Could you check a few things on this model? Use its own coordinates, in mm. Face numbers are marked on the shaded views. A direction names the side the tool comes from. Give positions to 0.01 mm unless a question says otherwise; leave off trailing zeros. Loops run counter-clockwise (first coordinate to the right, second up) from the corner with the lowest first, then second, coordinate; pieces in that order, holes last. Notation, with made-up numbers: (67, 57) - (96, 57) arc R21 ccw to (96, 96) - close; hole circle Ø7 at (39.25, 13). An arc over 180 degrees is marked (long way). Write each question's results on one line, items separated by ' | '. Start each with the question number.
(1) Suppose I cut it at B-B (y = 0). Please give me the cut outline in (x, z), and give its area (3 significant figures).
(2) Suppose I cut it at C-C (x = 43). Please give me the cut outline in (y, z).
(3) Suppose I cut it at A-A (x = 7.5). Please give me the cut outline in (y, z).
(4) If we mould it in two halves opening along X, with no side actions, what happens to the marked faces 3, 4 and 5? For each: released by +X, released by -X, zero draft, split by the parting line, or undercut.
(5) On a 3-axis mill with a long thin cutter (end or side, diameter ignored), from which of +Z, -Z, +X, -X, +Y, -Y can I reach the whole of each face in a straight line? I mean the marked faces 1 and 2. Say none if no direction works.
(6) I need wall thicknesses on line 1 (Y direction, x = -8, z = 3.75); line 2 (X direction, y = 30, z = 3.5); line 3 (Y direction, x = -45.5, z = 6.5). Which ranges of each line are inside material? Lowest first, please.
(7) Suppose I cut it at D-D (y = 15). Please give me the cut outline in (x, z), and give its area (3 significant figures).
(8) For pin 1 (5 mm diameter, centred on y = -44.5, z = 4.5, fed in from -X) (3 decimals); pin 2 (18 mm diameter, centred on x = -9.62, y = -27.94, fed in from +Z); pin 3 (4 mm diameter, centred on x = 29.5, z = 7.5, fed in from +Y); pin 4 (23 mm diameter, centred on x = 49.98, y = 0, fed in from +Z), each with a flat end and sliding along its axis, tell me the tip position at first contact or that it passes through.
from build123d import *

# Parameters (mm, degrees)
F0_R     = 12.7
F0_R_2   = 6.927169
F1_DEPTH = 12.7


with BuildPart() as f1:
    # F0 (on Top) → F1 (new body)
    with BuildSketch(Plane.XY):
        with BuildLine():
            Line((24.191197, 48.60003), (16.581545, 50.826576))
            ThreePointArc((16.581545, 50.826576), (-0.05997, 65.800738), (-17.259652, 51.47117))
            Line((-17.259652, 51.47117), (-24.214894, 47.664739))
            ThreePointArc((-24.214894, 47.664739), (-46.570553, 46.485742), (-48.60003, 24.191197))
            Line((-48.60003, 24.191197), (-50.826576, 16.581545))
            ThreePointArc((-50.826576, 16.581545), (-65.800738, -0.05997), (-51.47117, -17.259652))
            Line((-51.47117, -17.259652), (-47.664739, -24.214894))
            ThreePointArc((-47.664739, -24.214894), (-46.485742, -46.570553), (-24.191197, -48.60003))
            Line((-24.191197, -48.60003), (-16.581545, -50.826576))
            ThreePointArc((-16.581545, -50.826576), (0.05997, -65.800738), (17.259652, -51.47117))
            Line((17.259652, -51.47117), (24.214894, -47.664739))
            ThreePointArc((24.214894, -47.664739), (46.570553, -46.485742), (48.60003, -24.191197))
            Line((48.60003, -24.191197), (50.826576, -16.581545))
            ThreePointArc((50.826576, -16.581545), (65.800738, 0.05997), (51.47117, 17.259652))
            Line((51.47117, 17.259652), (47.664739, 24.214894))
            ThreePointArc((47.664739, 24.214894), (46.485742, 46.570553), (24.191197, 48.60003))
        make_face()
        with Locations((-35.343174, -35.343174)):
            Circle(F0_R, mode=Mode.SUBTRACT)
        with Locations((-9.619523, -27.942425)):
            Circle(F0_R_2, mode=Mode.SUBTRACT)
        with Locations((0, -49.982796)):
            Circle(F0_R, mode=Mode.SUBTRACT)
        with Locations((35.343174, -35.343174)):
            Circle(F0_R, mode=Mode.SUBTRACT)
        with Locations((27.942425, -9.619523)):
            Circle(F0_R_2, mode=Mode.SUBTRACT)
        with Locations((-49.982796, 0)):
            Circle(F0_R, mode=Mode.SUBTRACT)
        with Locations((-27.942425, 9.619523)):
            Circle(F0_R_2, mode=Mode.SUBTRACT)
        with Locations((-35.343174, 35.343174)):
            Circle(F0_R, mode=Mode.SUBTRACT)
        Circle(F0_R, mode=Mode.SUBTRACT)
        with Locations((9.619523, 27.942425)):
            Circle(F0_R_2, mode=Mode.SUBTRACT)
        with Locations((49.982796, 0)):
            Circle(F0_R, mode=Mode.SUBTRACT)
        with Locations((0, 49.982796)):
            Circle(F0_R, mode=Mode.SUBTRACT)
        with Locations((35.343174, 35.343174)):
            Circle(F0_R, mode=Mode.SUBTRACT)
    extrude(amount=F1_DEPTH)


solid = f1.part
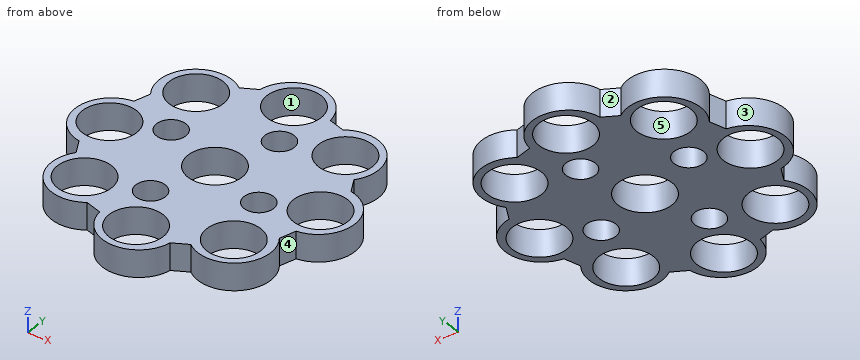
Output values:
1) outline: (-65.8, 0) - (-62.68, 0) - (-62.68, 12.7) - (-65.8, 12.7) - close; (-37.28, 0) - (-12.7, 0) - (-12.7, 12.7) - (-37.28, 12.7) - close; (12.7, 0) - (37.28, 0) - (37.28, 12.7) - (12.7, 12.7) - close; (62.68, 0) - (65.8, 0) - (65.8, 12.7) - (62.68, 12.7) - close | area: 704 mm2
2) outline: (-49.12, 0) - (-45.48, 0) - (-45.48, 12.7) - (-49.12, 12.7) - close; (-25.21, 0) - (-10.61, 0) - (-10.61, 12.7) - (-25.21, 12.7) - close; (10.61, 0) - (25.21, 0) - (25.21, 12.7) - (10.61, 12.7) - close; (45.48, 0) - (49.35, 0) - (49.35, 12.7) - (45.48, 12.7) - close
3) outline: (-64.25, 0) - (-60.23, 0) - (-60.23, 12.7) - (-64.25, 12.7) - close; (-39.73, 0) - (-10.25, 0) - (-10.25, 12.7) - (-39.73, 12.7) - close; (10.25, 0) - (21.35, 0) - (21.35, 12.7) - (10.25, 12.7) - close; (34.54, 0) - (39.73, 0) - (39.73, 12.7) - (34.54, 12.7) - close; (60.23, 0) - (63.88, 0) - (63.88, 12.7) - (60.23, 12.7) - close
4) face 3: released by -X | face 4: released by +X | face 5: undercut
5) face 1: +Z, -Z | face 2: +Z, -Z, +Y
6) line 1: -63.61 to -59.85, -40.12 to -34.68, -21.21 to -9.86, 9.86 to 40.12, 59.85 to 64.01 | line 2: -51.3 to -46.86, -23.82 to 3, 16.23 to 23.82, 46.86 to 50.6 | line 3: -47.52 to -42.97, -27.72 to -11.88, 11.88 to 27.72, 42.97 to 47.43
7) outline: (-56.17, 0) - (-32.31, 0) - (-32.31, 12.7) - (-56.17, 12.7) - close; (-23.58, 0) - (57.58, 0) - (57.58, 12.7) - (-23.58, 12.7) - close | area: 1,330 mm2
8) pin 1: x = -49.635 | pin 2: z = 12.7 | pin 3: y = 51.6 | pin 4: through
